Design review of the part shown in the three views and the two pictorial views. Dimensions are in mm from the part's minimum x, y and z. A direction names the side the tool comes from. Round coordinates to 2 decimals unless told otherwise and drop trailing zeros. Write each loop counter-clockwise with the first axis right and the second up, starting at its lowest first coordinate (ties: lowest second). Pieces come first, ordered by that corner, then holes. Notation, with made-up numbers: (13.5, -7.75) - (69.5, -7.75) arc R27 cw to (69.5, 18.25) - close; hole circle Ø8 at (3.5, -24.5). An arc over 180 degrees is marked (long way). Use one line per item in the form item = value.
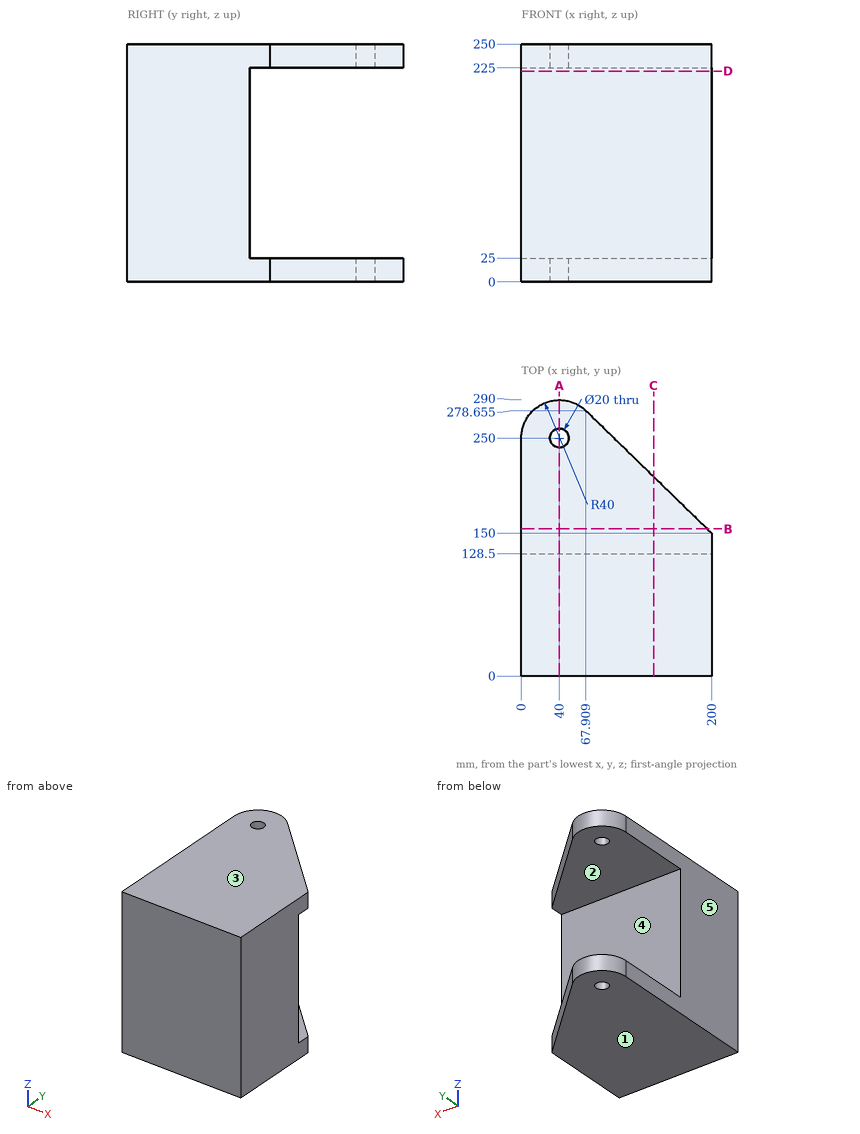
Q1. We need section D-D on z = 221.5. Write out the cut boundary in (x, y).
Calculated:
outline = (0, 0) - (200, 0) - (200, 128.5) - (0, 128.5) - close
Q2. We need section A-A on x = 40. Write out the cut boundary in (y, z).
Calculated:
outline = (0, 0) - (240, 0) - (240, 25) - (128.5, 25) - (128.5, 225) - (240, 225) - (240, 250) - (0, 250) - close; (260, 0) - (290, 0) - (290, 25) - (260, 25) - close; (260, 225) - (290, 225) - (290, 250) - (260, 250) - close
Q3. For P1, Ø8, axis at x = 141.5, z = 27.5, coming from the +Y side; P2, Ø1, axis at x = 152.5, z = 51.5, coming from the -Y side; P3, Ø5, axis at x = 56, z = 160.5, coming from the +Y side, all flat-tipped, find the tip position at first contact; note any pin that passes through.
Calculated:
P1 = 210.02
P2 = 0
P3 = 128.5
Q4. Machinability: for the marked faces 1 and 2, which of the approach directions +Z, -Z, +X, -X, +Y, -Y give a long, thin tool a straight path to every point of the face, cutting with its end or side? Answer none if there is none.
Calculated:
face_1 = -Z, +X, -X, +Y, -Y
face_2 = +X, -X, +Y
Q5. We need section B-B on y = 154.5. Write out the cut boundary in (x, z).
Calculated:
outline = (0, 0) - (195.38, 0) - (195.38, 25) - (0, 25) - close; (0, 225) - (195.38, 225) - (195.38, 250) - (0, 250) - close
Q6. To check wall thickness, follow line 1 along Z through (x, y) = (159, 174); line 2 along Y through (x, z) = (40, 237.25); line 3 along Y through (x, z) = (167, 67). State the ranges of each line that lie inside material, in increasing order. Write a range as from..to.
Calculated:
line_1 = 0..25, 225..250
line_2 = 0..240, 260..290
line_3 = 0..128.5
Q7. Draft analysis for pull direction Z (two halves, no side actions). For the marked faces 3, 4 and 5, state which applies: released by +Z, released by -Z, zero draft, split by the parting line, or undercut.
Calculated:
face_3 = released by +Z
face_4 = undercut
face_5 = zero draft
Q8. We need section C-C on x = 139. Write out the cut boundary in (y, z).
Calculated:
outline = (0, 0) - (209.41, 0) - (209.41, 25) - (128.5, 25) - (128.5, 225) - (209.41, 225) - (209.41, 250) - (0, 250) - close
